Geometry check sheet. Reference: the model listing, model coordinates, mm. A direction names the side the tool comes from. Round coordinates to 2 decimals unless told otherwise and drop trailing zeros. Order: outer loops, then holes, each group sorted by start corner. A loop starts at its lowest first (then second) coordinate and runs counter-clockwise, first axis right, second up. Notation, with made-up numbers: (11, 59.25) - (69, 59.25) arc R10 ccw to (69, 78.25) - close; hole circle Ø8 at (42, -11). An arc over 180 degrees is marked (long way). One line per question, with ' | ' between items. Start each with the question number.
Q1. Material ranges on line 1 along X through (y, z) = (3513, 2.25); line 2 along Y through (x, z) = (6278, 1.6); line 3 along X through (y, z) = (3557.5, 0.25), recorded low to high.
Q2. Mould release check, pull along X, two halves, no side actions. Record for faces 5 (the face through (6280.038, 3497.577, 1.678)), 6 (the face through (6281.518, 3512.354, 1.678)), 7 (the face through (6342.809, 3559.643, 1.678)), 8 (the face through (6259, 3499.784, 2)): +X half, -X half, draft (parallel to the pull), parting line (faces both ways), or undercut.
Q3. Sectioned sample at A-A, the plane y = 3553. Enter the section's corners in (x, z).
Q4. Sectioned sample at B-B, the plane x = 6341.5. Enter the section's corners in (y, z), then the cut area to 3 significant figures.
Q5. Tool access check on faces 1 (the face through (6357.47, 3569, 2)), 2 (the face through (6296.765, 3504.402, 1.678)), 3 (the face through (6259, 3570.751, 2)), 4 (the face through (6354, 3563.081, 2)). Record the directions out of +Z, -Z, +X, -X, +Y, -Y that give a thin tool (end or side, any length) a straight path to the whole face; none if there is none.
Q6. Sectioned sample at C-C, the plane x = 6278.5. Enter the section's corners in (y, z).
Q7. Gauge pin test, flat ends, axial feed: P1, Ø1.7, axis at y = 3536, z = 1.5, coming from the -X side; P2, Ø1.7, axis at x = 6306.5, z = 2, coming from the +Y side; P3, Ø1, axis at x = 6257, z = 1, coming from the -Y side. Record the tip position at first contact, or that the pin passes through.
Q8. Sectioned sample at D-D, the plane y = 3524.5. Enter the section's corners in (x, z).
```python
from build123d import *

# Parameters (mm, degrees)
SKETCH1_R           = 2.921000021
BOSS_EXTRUDE1_DEPTH = 3.4036


with BuildPart() as part:
    # Sketch1 → Boss-Extrude1 (new body)
    with BuildSketch(Plane.XY):
        Polygon((6298.761762124, 3495.306881262), (6321.380962278, 3495.307266858), (6357.4701776, 3494.754624258), (6357.4701776, 3507.454624258), (6350.731610594, 3507.454624258), (6350.731610594, 3563.080624258), (6357.4701776, 3563.080624258), (6357.4701776, 3575.780624258), (6321.380962278, 3575.227981658), (6298.761762124, 3575.228367254), (6261.831610594, 3570.751424258), (6255.481610594, 3570.751424258), (6255.481610594, 3558.051424258), (6261.831610594, 3558.051424258), (6261.831610594, 3512.483824258), (6255.481610594, 3512.483824258), (6255.481610594, 3499.783824258), (6261.831610594, 3499.783824258), align=None)
        with Locations((6278.820230754, 3513.47268496)):
            Circle(SKETCH1_R, mode=Mode.SUBTRACT)
        with Locations((6341.280374087, 3513.414361889)):
            Circle(SKETCH1_R, mode=Mode.SUBTRACT)
        with Locations((6341.23876101, 3557.180196157)):
            Circle(SKETCH1_R, mode=Mode.SUBTRACT)
        with Locations((6278.860987901, 3557.120886627)):
            Circle(SKETCH1_R, mode=Mode.SUBTRACT)
        with BuildLine():
            Line((6343.460429176, 3531.918193441), (6343.460314953, 3538.618193502))
            ThreePointArc((6343.460314953, 3538.618193502), (6342.349105565, 3541.300760923), (6339.666500257, 3542.411878844))
            Line((6339.666500257, 3542.411878844), (6336.09539352, 3542.411817963))
            ThreePointArc((6336.09539352, 3542.411817963), (6293.858290099, 3556.842691981), (6295.967723135, 3512.258240403))
            Line((6295.967723135, 3512.258240403), (6295.96782376, 3506.355583647))
            ThreePointArc((6295.96782376, 3506.355583647), (6296.78612787, 3504.380118018), (6298.761621398, 3503.561881261))
            Line((6298.761621398, 3503.561881261), (6298.761675524, 3500.386881261))
            Line((6298.761675524, 3500.386881261), (6321.380875678, 3500.387266857))
            Line((6321.380875678, 3500.387266857), (6321.380821552, 3503.562266857))
            ThreePointArc((6321.380821552, 3503.562266857), (6323.356287182, 3504.380570967), (6324.174523939, 3506.356064496))
            Line((6324.174523939, 3506.356064496), (6324.174423315, 3512.258721235))
            ThreePointArc((6324.174423315, 3512.258721235), (6331.646301452, 3519.055968956), (6336.095637085, 3528.124317864))
            Line((6336.095637085, 3528.124317864), (6339.666743834, 3528.124378745))
            ThreePointArc((6339.666743834, 3528.124378745), (6342.349311255, 3529.235588133), (6343.460429176, 3531.918193441))
        make_face(mode=Mode.SUBTRACT)
    extrude(amount=BOSS_EXTRUDE1_DEPTH)


solid = part.part
```
Determined:
1) line 1: x = 6261.83 to 6275.94, 6281.7 to 6294.82, 6325.32 to 6338.39, 6344.17 to 6350.73 | line 2: y = 3497.82 to 3510.67, 3516.28 to 3554.33, 3559.91 to 3572.71 | line 3: x = 6261.83 to 6275.96, 6281.76 to 6294.77, 6325.37 to 6338.34, 6344.14 to 6350.73
2) face 5: -X half | face 6: undercut | face 7: undercut | face 8: draft
3) outline: (6261.83, 0) - (6289.73, 0) - (6289.73, 3.4) - (6261.83, 3.4) - close; (6330.41, 0) - (6350.73, 0) - (6350.73, 3.4) - (6330.41, 3.4) - close
4) outline: (3495, 0) - (3510.5, 0) - (3510.5, 3.4) - (3495, 3.4) - close; (3516.33, 0) - (3528.6, 0) - (3528.6, 3.4) - (3516.33, 3.4) - close; (3541.94, 0) - (3554.27, 0) - (3554.27, 3.4) - (3541.94, 3.4) - close; (3560.09, 0) - (3575.54, 0) - (3575.54, 3.4) - (3560.09, 3.4) - close | area: 189 mm2
5) face 1: +Z, -Z, +X, +Y, -Y | face 2: +Z, -Z | face 3: +Z, -Z, -X, +Y | face 4: +Z, -Z, +X
6) outline: (3497.76, 0) - (3510.57, 0) - (3510.57, 3.4) - (3497.76, 3.4) - close; (3516.38, 0) - (3554.22, 0) - (3554.22, 3.4) - (3516.38, 3.4) - close; (3560.02, 0) - (3572.77, 0) - (3572.77, 3.4) - (3560.02, 3.4) - close
7) P1: stops at x = 6261.83 | P2: stops at y = 3575.23 | P3: stops at y = 3499.78
8) outline: (6261.83, 0) - (6285.32, 0) - (6285.32, 3.4) - (6261.83, 3.4) - close; (6334.82, 0) - (6350.73, 0) - (6350.73, 3.4) - (6334.82, 3.4) - close
